Model file for the job. Use its own axes, mm. Face numbers are marked on the shaded views. Coordinates: 2 decimals unless noted, no trailing zeros. Write each loop counter-clockwise with the first axis right and the second up, starting at its lowest first coordinate (ties: lowest second). Pieces come first, ordered by that corner, then holes. Notation, with made-up numbers: M 51.5,-33 L 78.5,-33 A22 cw 78.5,-7 Z; hole C 66.5,39.25 d7. An arc over 180 degrees is marked long. Answer in a Markdown table with one row per item. Add a question column.
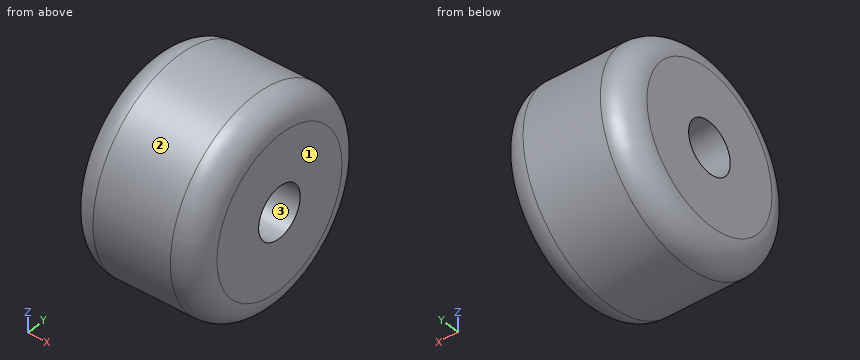
Autodesk Fusion 360 part; units mm, degrees
sketch "Sketch1" plane through (0, 0, 0) normal (1, 0, 0) x (0, 1, 0)
  circle A0 centre (0, 0) radius 1
  circle A1 centre (0, 0) radius 4
  dimension "d1" = 2
  dimension "d2" = 8
extrude "Extrude1" add sketch "Sketch1" along normal blind 5
fillet "Fillet1" radius 1 1 edges at (0, -3.7293, -1.4465)
fillet "Fillet2" radius 1 1 edges at (5, -3.7293, -1.4465)
1) Two-plate mould, pull along Y, no slides. Class the marked faces 1, 2 and 3: released by +Y, released by -Y, zero draft, split by the parting line, or undercut.
2) Drill centre lines: probe 1 along Z at (x, y) = (3.7, 0); probe 2 along Y at (x, z) = (2.95, -0.75); probe 3 along Y at (x, z) = (4.4, 3.5). Where is each one in solid material? Low to high.
3) Slice it at C-C (x = 1.8). Give the cut face in (y, z), then the cut area to 3 significant figures.
4) Slice it at A-A (y = 0). Give the cut face in (x, z).
Ans:
| question | item | result |
|---|---|---|
| 1 | face 1 | zero draft |
| 1 | face 2 | split by the parting line |
| 1 | face 3 | undercut |
| 2 | probe 1 | z = -4 to -1, 1 to 4 |
| 2 | probe 2 | y = -3.93 to -0.66, 0.66 to 3.93 |
| 2 | probe 3 | y = -1.76 to 1.76 |
| 3 | outline | C 0,0 d8; hole C 0,0 d2 |
| 3 | area | 47.1 mm2 |
| 4 | outline | M 0,-3 A1 ccw 1,-4 L 4,-4 A1 ccw 5,-3 L 5,-1 L 0,-1 Z; M 0,1 L 5,1 L 5,3 A1 ccw 4,4 L 1,4 A1 ccw 0,3 Z |
